Autodesk Inventor part; units mm, degrees
ref_plane "Work Plane1" through (0, 0, -15) normal (0, 0, 1) x (1, 0, 0)
ref_plane "YZ Plane" through (0, 0, 0) normal (1, 0, 0) x (0, 1, 0)
ref_plane "XZ Plane" through (0, 0, 0) normal (0, 1, 0) x (-1, 0, 0)
sketch "Sketch1" plane through (0, 0, 0) normal (0, 0, 1) x (1, 0, 0)
  line L0 (0, 0) -> (25, 0)
  line L1 (25, 0) -> (25, 40)
  line L2 (25, 40) -> (0, 40)
  line L3 (0, 40) -> (0, 0)
  dimension "d1" = 25
  dimension "d2" = 40
  dimension "d3" = 25
extrude "Extrusion1" add sketch "Sketch1" against normal blind 30
sketch "Sketch2" plane through (25, 0, 0) normal (1, 0, 0) x (0, 0, -1)
  line L0 (0, 0) -> (30, 0)
  circle A0 centre (15, 6.56) radius 2.46
extrude "Extrusion2" cut sketch "Sketch2" against normal blind 30
sketch "Sketch3" plane through (0, 0, 0) normal (-1, 0, 0) x (0, 0, 1)
  line L0 (0, 0) -> (-30, 0)
  line L1 (-25.05, 0) -> (-4.95, 0)
  line L2 (-4.95, 0) -> (-4.95, 33.12)
  line L3 (-4.95, 33.12) -> (-25.05, 33.12)
  line L4 (-25.05, 33.12) -> (-25.05, 0)
  dimension "d11" = 20.1
extrude "Extrusion3" cut sketch "Sketch3" against normal blind 20
sketch "Sketch4" plane through (0, 0, 0) normal (0, -1, 0) x (1, 0, 0)
  line L0 (20, -4.95) -> (20, -25.05)
  line L1 (20, -15) -> (25, -15)
  line L2 (25, 0) -> (25, -30)
  line L3 (20, -8.025) -> (25, -8.025)
  line L4 (25, -8.025) -> (25, -21.975)
  line L5 (25, -21.975) -> (20, -21.975)
  line L6 (20, -21.975) -> (20, -8.025)
  line L7 (20, -8.025) -> (25, -21.975) construction
  line L8 (25, -8.025) -> (20, -21.975) construction
  line L9 (25, -12.54) -> (25, -17.46)
  point P0 (0, 0)
  point P1 (22.5, -15)
  dimension "d14" = 13.95
extrude "Extrusion4" add sketch "Sketch4" along normal blind 15
sketch "Sketch5" plane through (20, 0, 0) normal (-1, 0, 0) x (0, 0, 1)
  circle A0 centre (-15, 6.56) radius 2.46
  circle A1 centre (-15, 6.56) radius 4.7025
  circle A2 centre (-15, 6.56) radius 2.46
  circle A3 centre (-15, 6.56) radius 2.46
  point P0 (0, 0)
  dimension "d17" = 9.405
extrude "Extrusion5" cut sketch "Sketch5" against normal blind 2.1
sketch "Sketch6" plane through (25, 0, 0) normal (1, 0, 0) x (0, 0, -1)
  circle A0 centre (15, 6.56) radius 4.7025
  line L0 (15, 6.56) -> (15, 23.56)
  circle A1 centre (15, 23.56) radius 2.46
  point P0 (0, 0)
  dimension "d20" = 17
  dimension "d21" = 4.92
extrude "Extrusion6" cut sketch "Sketch6" against normal blind 10 contours A1
sketch "Sketch7" plane through (20, 0, 0) normal (-1, 0, 0) x (0, 0, 1)
  circle A0 centre (-15, 23.56) radius 2.46
  circle A1 centre (-15, 23.56) radius 4.7025
  point P0 (0, 0)
  dimension "d24" = 9.405
extrude "Extrusion7" cut sketch "Sketch7" against normal blind 2.1
sketch "Sketch9" plane through (25, 0, 0) normal (1, 0, 0) x (0, 0, -1)
  circle A0 centre (15, 6.56) radius 2.46
  circle A1 centre (15, 6.56) radius 2.46
  circle A2 centre (15, 23.56) radius 2.46
  circle A3 centre (15, 23.56) radius 2.46
  line L0 (30, 40) -> (30, 0)
  line L1 (30, 0) -> (30, 40)
  line L2 (30, 40) -> (0, 40)
  line L3 (0, 40) -> (0, 0)
  line L4 (0, 0) -> (8.025, 0)
  line L5 (21.975, 0) -> (21.975, -15)
  line L6 (21.975, -15) -> (8.025, -15)
  line L7 (8.025, -15) -> (8.025, 0)
  line L8 (0, 0) -> (8.025, 0)
  line L9 (21.975, 0) -> (30, 0)
extrude "Extrusion8" add sketch "Sketch9" along normal blind 5
sketch "Sketch10" plane through (0, 40, 0) normal (0, 1, 0) x (1, 0, 0)
  line L0 (0, 30) -> (30, 30)
  line L1 (30, 0) -> (0, 0)
  line L2 (0, 30) -> (30, 30)
  line L3 (30, 30) -> (30, 0)
  line L4 (30, 0) -> (0, 0)
  line L5 (0, 0) -> (0, 30)
extrude "Extrusion9" add sketch "Sketch10" along normal blind 30
sketch "Sketch12" plane through (30, 0, 0) normal (1, 0, 0) x (0, 0, -1)
  circle A0 centre (15, 6.56) radius 2.46
  line L0 (15, 6.56) -> (15, 15.06)
  circle A1 centre (15, 15.06) radius 2.525
  point P0 (0, 0)
  dimension "d31" = 8.5
  dimension "d33" = 5.05
extrude "Extrusion10" cut sketch "Sketch12" against normal blind 30 contours A1
sketch "Sketch14" plane through (0, 0, 0) normal (0, 0, 1) x (1, 0, 0)
  line L0 (30, 70) -> (0, 70)
  line L1 (0, 100) -> (-8, 100)
  line L2 (30, 0) -> (30, 70)
  line L3 (30, 118) -> (30, 70)
  line L4 (30, 105) -> (30, 100)
  line L5 (-2, 134) -> (-8, 136)
  line L6 (-2, 134) -> (4, 118)
  line L7 (-2, 102) -> (-8, 100)
  line L8 (-2, 102) -> (4, 118)
  line L9 (0, 70) -> (30, 70)
  line L10 (0, 70) -> (0, 100)
  line L11 (15, 136) -> (30, 118)
  line L12 (-8, 136) -> (15, 136)
  point P0 (0, 0)
  dimension "d47" = 30
extrude "Extrusion12" add sketch "Sketch14" against normal blind 30
sketch "Sketch15" plane through (0, 0, -25.05) normal (-1, 0, 0) x (0, 0, 1)
  line L0 (0, 33.12) -> (20.1, 33.12)
  line L1 (20.1, 33.12) -> (20.1, 0)
  line L2 (0, 33.12) -> (20.1, 33.12)
  line L3 (20.1, 33.12) -> (20.1, 31.1)
  line L4 (20.1, 31.1) -> (0, 31.1)
  line L5 (0, 31.1) -> (0, 33.12)
  point P0 (25.05, 0)
  dimension "d57" = 2.02
extrude "Extrusion13" add sketch "Sketch15" against normal blind 20
sketch "Sketch23" plane through (0, 0, 0) normal (0, 0, 1) x (1, 0, 0)
  line L0 (0, 100) -> (-8, 100)
  line L1 (-8, 100) -> (-2, 102)
  line L2 (-8, 100) -> (-2, 102)
  line L3 (-2, 102) -> (4, 118)
  line L4 (-2, 102) -> (4, 118)
  line L5 (-2, 134) -> (4, 118)
  line L6 (4, 118) -> (-2, 134)
  line L7 (-2, 134) -> (-8, 136)
  line L8 (-2, 134) -> (-8, 136)
  line L9 (-8, 136) -> (15, 136)
  line L10 (-8, 136) -> (15, 136)
  line L11 (30, 118) -> (15, 136)
  line L12 (15, 136) -> (30, 118)
  line L13 (30, 118) -> (30, 93)
  line L14 (30, 0) -> (30, 118)
  line L15 (30, 93) -> (0, 93)
  line L16 (0, 93) -> (0, 100)
  line L17 (-8, 100) -> (0, 100)
  point P0 (0, 0)
  dimension "d85" = 25
extrude "Extrusion14" add sketch "Sketch23" along normal blind 15
ref_plane "Work Plane1" through (0, 0, -15) normal (0, 0, 1) x (1, 0, 0)
mirror "Mirror1" about plane through (0, 0, -15) normal (0, 0, 1) of "Extrusion14"
properties part number "32mm_x_60mm"
For this review, take the finished solid that the model builds, in its own axes (mm). A direction names the side the tool comes from. Round coordinates to 2 decimals unless told otherwise and drop trailing zeros. Order: outer loops, then holes, each group sorted by start corner. A loop starts at its lowest first (then second) coordinate and runs counter-clockwise, first axis right, second up. Notation, with made-up numbers: M -11,85 L 21,85 A18 cw 21,105 Z; hole C -21.75,47 d4. An arc over 180 degrees is marked long. Write each question's results on one line, items separated by ' | '. Start each with the question number.
1. Tool access review of faces 5 (the face through (-5, 135, -15)), 6 (the face through (10, 16, -25.05)), 7 (the face through (15, 47, 0)), 8 (the face through (0, 62, -15)): name each direction out of +Z, -Z, +X, -X, +Y, -Y from which nothing blocks a thin tool from reaching the whole face with its end or side.
2. Add section B-B (z = -15). State how many separate pieces and enclosed holes the cut face has, then the cut area to 3 significant figures.
3. Clearance check with flat-ended pins moving along their axes: pin 1 Ø3 at (y, z) = (48.5, -17) entering from -X; pin 2 Ø1.5 at (x, z) = (10.5, -13.5) entering from -Y; pin 3 Ø6 at (x, y) = (24, 87) entering from +Z. State where each tip first meets the part, or that it passes through.
4. To check wall thickness, follow L1, parallel to Z at x = 8.5, y = 4.5; L2, parallel to Y at x = 24, z = -15 (3 decimals); L3, parallel to Y at x = 26, z = -15 (3 decimals). State the ranges of each line that lie inside material, in increasing order. Write a range as [from, to].
5. Add section A-A (y = 15.06). State the section outline as (x, z) points (3 decimals), then the cut area to 4 significant figures.
6. Add section C-C (z = -40). State the section outline as (x, y) points.
7. Add section D-D (x = 10.5). State the section outline as (y, z) points, then the cut area to 3 significant figures.
8. Draft analysis for pull direction Z (two halves, no side actions). For faces 1 (the face through (25, -8, -8.025)), 2 (the face through (15, 93, 7)), 3 (the face through (15, 115, -45)), 4 (the face through (22.1, 4.5, -13)), state which applies: pulls with the +Z half, pulls with the -Z half, needs draft (parallel to the pull), parting line crosses it, or undercut.
Output values:
1) face 5: +Z, -Z, -X | face 6: -X, -Y | face 7: +Z, +X, -X, -Y | face 8: +Z, -Z, -X, -Y
2) separate pieces: 4 | enclosed holes: 0 | area: 3,290 mm^2
3) pin 1: x = 0 | pin 2: y = 31.1 | pin 3: z = 0
4) L1: [-30, -25.05], [-4.95, 0] | L2: [-15, 4.1], [9.02, 12.535], [17.585, 21.1], [26.02, 125.2] | L3: [-15, 4.1], [9.02, 12.535], [17.585, 21.1], [26.02, 122.8]
5) outline: M 0,-30 L 30,-30 L 30,-17.525 L 20,-17.525 L 20,-25.05 L 0,-25.05 Z; M 0,-4.95 L 20,-4.95 L 20,-12.475 L 30,-12.475 L 30,0 L 0,0 Z | area: 447.5 mm^2
6) outline: M -8,100 L 0,100 L 0,93 L 30,93 L 30,118 L 15,136 L -8,136 L -2,134 L 4,118 L -2,102 Z
7) outline: M 0,-30 L 93,-30 L 93,-45 L 136,-45 L 136,15 L 93,15 L 93,0 L 0,0 L 0,-4.95 L 31.1,-4.95 L 31.1,-25.05 L 0,-25.05 Z | area: 4,740 mm^2
8) face 1: pulls with the +Z half | face 2: needs draft | face 3: pulls with the -Z half | face 4: undercut
